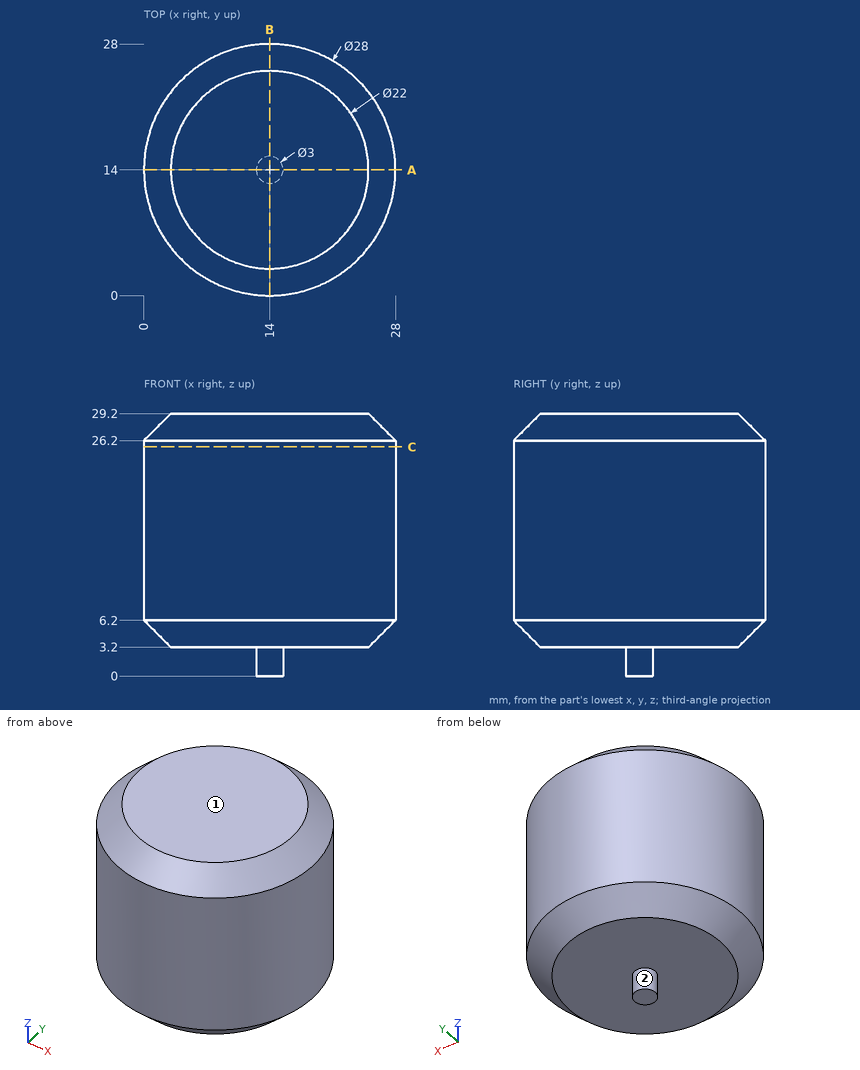
Geometry check sheet. Reference: drawing and pictorial views, mm from the part's lowest x, y, z. A direction names the side the tool comes from. Give positions to 0.01 mm unless a question says otherwise; leave off trailing zeros. Order: outer loops, then holes, each group sorted by start corner. A loop starts at its lowest first (then second) coordinate and runs counter-clockwise, first axis right, second up. Notation, with made-up numbers: (67, 63) -> (126, 63) arc R4 cw to (126, 67) -> close; hole circle Ø5 at (47, 40.25). An arc over 180 degrees is marked (long way). Use CSV: the item, a comma, the result in double quotes. Start each with the question number.
1) Material ranges on line 1 (Z direction, x = 17.5, y = 17.75); line 2 (Y direction, x = 14.25, z = 25.5); line 3 (Y direction, x = 23.25, z = 13), recorded low to high. Write a range as from..to.
2) Set-up check for the marked faces 1 and 2: record each of +Z, -Z, +X, -X, +Y, -Y from which the full face is reachable in a straight line by a thin tool's end or side.
3) Go/stop test with flat-tipped pins: P1, Ø6, axis at y = 3.5, z = 19, coming from the -X side; P2, Ø2, axis at y = 19, z = 8.5, coming from the -X side; P3, Ø2, axis at x = 9.5, y = 24.5, coming from the -Z side. Record where each tip stops, or that it passes through.
4) Sectioned sample at A-A, the plane y = 14. Record the boundary of the cut face in (x, z).
5) Sectioned sample at C-C, the plane z = 25.5. Record the boundary of the cut face in (x, y).
Recorded:
1,line 1,"3.2..29.2"
1,line 2,"0..28"
1,line 3,"3.49..24.51"
2,face 1,"+Z, +X, -X, +Y, -Y"
2,face 2,"-Z"
3,P1,"x = 2.18"
3,P2,"x = 0.58"
3,P3,"z = 3.2"
4,outline,"(0, 6.2) -> (3, 3.2) -> (12.5, 3.2) -> (12.5, 0) -> (15.5, 0) -> (15.5, 3.2) -> (25, 3.2) -> (28, 6.2) -> (28, 26.2) -> (25, 29.2) -> (3, 29.2) -> (0, 26.2) -> close"
5,outline,"circle Ø28 at (14, 14)"
